```python
from build123d import *

# Parameters (mm, degrees)
BOSS_EXTRUDE2_DEPTH = 7.62


with BuildPart() as part:
    # Sketch1 → Boss-Extrude2 (new body)
    with BuildSketch(Plane.XY):
        with BuildLine():
            Line((8.798818102, -5.08), (91.44451632, -5.08))
            ThreePointArc((91.44451632, -5.08), (110.403219868, 0.048246477), (91.396667211, 4.996206486))
            Line((91.396667211, 4.996206486), (8.846667211, 4.996206486))
            ThreePointArc((8.846667211, 4.996206486), (1.926604894, 9.975660057), (-6.35, 7.931147458))
            Line((-6.35, 7.931147458), (-6.35, 6.35))
            Line((-6.35, 6.35), (0, 6.35))
            Line((0, 6.35), (3.81, 0))
            Line((3.81, 0), (0, -6.35))
            Line((0, -6.35), (-6.35, -6.35))
            Line((-6.35, -6.35), (-6.35, -7.931147458))
            ThreePointArc((-6.35, -7.931147458), (1.879212064, -9.984696391), (8.798818102, -5.08))
        make_face()
        Polygon((96.577160213, 6.35), (103.909508632, 6.35), (107.575682841, 0), (103.909508632, -6.35), (96.577160213, -6.35), (92.910986004, 0), align=None, mode=Mode.SUBTRACT)
    extrude(amount=BOSS_EXTRUDE2_DEPTH)


solid = part.part
```
Work out the finished part from the listing and answer in its coordinate system (mm). A direction names the side the tool comes from. Give positions to 0.01 mm unless a question says otherwise; leave off trailing zeros. Write each loop counter-clockwise with the first axis right and the second up, starting at its lowest first coordinate (ties: lowest second). Pieces come first, ordered by that corner, then holes. Notation, with made-up numbers: (7.5, -38.5) -> (24.5, -38.5) arc R27 ccw to (24.5, -13.5) -> close; hole circle Ø2 at (20.25, 47.25). An arc over 180 degrees is marked (long way). Write each question's results on one line, items separated by ' | '.
1. A tool of negligible diameter and unlimited length cuts with its end or side. For faces 4 (the cylindrical face through (1.8, -10, 3.8)), 5 (the flat face through (-3, 6.35, 4)), 6 (the flat face through (51, 4.996, 4)), 7 (the flat face through (94.77, -3.22, 3.76)), from which of +Z, -Z, +X, -X, +Y, -Y can it reach the whole face along a straight path? Write none if from no direction.
Data:
face 4: +Z, -Z, -Y | face 5: +Z, -Z, -X | face 6: +Z, -Z, +Y | face 7: +Z, -Z
2. Find section B-B on y = 2.75. Determine the outline of the cut face in (x, z).
Data:
outline: (2.16, 0) -> (94.5, 0) -> (94.5, 7.62) -> (2.16, 7.62) -> close; (105.99, 0) -> (110.02, 0) -> (110.02, 7.62) -> (105.99, 7.62) -> close
3. Determine the mould class of faces 1 (the flat face through (51, 0, 0)), 2 (the flat face through (50, -5.08, 4)), 3 (the flat face through (1.88, 3.22, 3.76)) for opening direction X: +X half, -X half, draft (parallel to the pull), parting line (faces both ways), or undercut.
Data:
face 1: draft | face 2: undercut | face 3: -X half
4. Straight lines are drawn through the part: L1, parallel to Y at x = 100, z = 2.5; L2, parallel to Y at x = 57.5, z = 5.75; L3, parallel to X at y = 0, z = 3.5. For each, find the intervals that lie inside material, in ascending order.
Data:
L1: -10.16 to -6.35, 6.35 to 10.16 | L2: -5.08 to 5 | L3: 3.81 to 92.91, 107.58 to 110.4
5. Find section A-A on z = 3.5. Determine the outline of the cut face in (x, y), and give its area (3 significant figures).
Data:
outline: (-6.35, -7.93) arc R10.16 ccw to (8.8, -5.08) -> (91.44, -5.08) arc R10.16 ccw (long way) to (91.4, 5) -> (8.85, 5) arc R10.16 ccw to (-6.35, 7.93) -> (-6.35, 6.35) -> (0, 6.35) -> (3.81, 0) -> (0, -6.35) -> (-6.35, -6.35) -> close; hole (92.91, 0) -> (96.58, -6.35) -> (103.91, -6.35) -> (107.58, 0) -> (103.91, 6.35) -> (96.58, 6.35) -> close | area: 1,180 mm^2
6. Find section C-C on x = 78. Determine the outline of the cut face in (y, z).
Data:
outline: (-5.08, 0) -> (5, 0) -> (5, 7.62) -> (-5.08, 7.62) -> close
7. Each of these flat-tipped pins is pushed along its axis until it touches: pin 1 Ø4 at (y, z) = (4, 1) entering from -X; pin 2 Ø1.9 at (x, z) = (-3.5, 5) entering from -Y; pin 3 Ø5 at (x, y) = (84.5, -4) entering from -Z; pin 4 Ø3 at (y, z) = (-5.5, 5) entering from +X. Where does it stop, or does it pass through?
Data:
pin 1: x = 0.21 | pin 2: y = -9.83 | pin 3: z = 0 | pin 4: x = 109.58
